For this review, take the finished solid that the model builds, in its own axes (mm). Face numbers are marked on the shaded views. A direction names the side the tool comes from. Give positions to 0.01 mm unless a question says otherwise; leave off trailing zeros. Write each loop counter-clockwise with the first axis right and the second up, starting at its lowest first coordinate (ties: lowest second). Pieces come first, ordered by that corner, then holes. Notation, with made-up numbers: M -3.75,-13 L 24.25,-13 A17 cw 24.25,3 Z; hole C 19,68.5 d6. An arc over 180 degrees is marked long. One line per item, written item: value. Start each with the question number.
Item 1: To check wall thickness, follow probe 1 along Y at (x, z) = (8.5, -13); probe 2 along Y at (x, z) = (26, 10); probe 3 along Z at (x, y) = (-8.5, 2) (3 decimals). State the ranges of each line that lie inside material, in increasing order.
Item 2: Consider section B-B, the plane z = 3. Write out the cut boundary in (x, y), and give its area (3 significant figures).
Item 3: Tool access review of the marked faces 1 and 2: name each direction out of +Z, -Z, +X, -X, +Y, -Y from which nothing blocks a thin tool from reaching the whole face with its end or side.
Item 4: Clearance check with flat-ended pins moving along their axes: pin 1 Ø0.6 at (y, z) = (3, 6.5) entering from +X; pin 2 Ø1 at (x, z) = (3.5, -11) entering from +Y; pin 3 Ø2.5 at (x, z) = (29, -11.875) entering from -Y. State where each tip first meets the part, or that it passes through.
Item 5: Consider section C-C, the plane y = -0.75. Write out the cut boundary in (x, z) (3 decimals), and give its area (3 significant figures).
Item 6: Consider section A-A, the plane x = -0.5. Write out the cut boundary in (y, z) (3 decimals), and give its area (3 significant figures).
```python
from build123d import *

# Parameters (mm, degrees)
EXTRUDE_1_DEPTH     = 1.63
SKETCH_2_R          = 1.5
CUT_EXTRUDE_1_DEPTH = 1.6
SKETCH_3_W          = 26.5
SKETCH_3_H          = 26
EXTRUDE_2_DEPTH     = 1.8
EXTRUDE_3_DEPTH     = 2
SKETCH_4_W          = 5.81
SKETCH_4_H          = 3.67
EXTRUDE_4_DEPTH     = 2
SKETCH_7_W          = 2.6
SKETCH_7_H          = 1.3
EXTRUDE_5_DEPTH     = 1
SKETCH_8_W          = 51
SKETCH_8_H          = 5
EXTRUDE_6_DEPTH     = 3.68
SKETCH_9_W          = 1.9
SKETCH_9_H          = 1.9
EXTRUDE_7_DEPTH     = 3
SKETCH_10_R         = 1.6
EXTRUDE_8_DEPTH     = 1


with BuildPart() as part:
    # 草图1 → 凸台-拉伸1 (new body)
    with BuildSketch(Plane(origin=(0, 0, 0), x_dir=(1, 0, 0), z_dir=(0, 1, 0))):
        with BuildLine():
            Line((-29.5, 15.375), (29.5, 15.375))
            ThreePointArc((29.5, 15.375), (31.621320344, 14.496320344), (32.5, 12.375))
            Line((32.5, 12.375), (32.5, -12.375))
            ThreePointArc((32.5, -12.375), (31.621320344, -14.496320344), (29.5, -15.375))
            Line((29.5, -15.375), (-29.5, -15.375))
            ThreePointArc((-29.5, -15.375), (-31.621320344, -14.496320344), (-32.5, -12.375))
            Line((-32.5, -12.375), (-32.5, 12.375))
            ThreePointArc((-32.5, 12.375), (-31.621320344, 14.496320344), (-29.5, 15.375))
        make_face()
    extrude(amount=EXTRUDE_1_DEPTH)

    # 草图2 → 切除-拉伸1 (cut)
    with BuildSketch(Plane(origin=(0, 1.63, 0), x_dir=(1, 0, 0), z_dir=(0, 1, 0))):
        with Locations(Location((-29, 11.875, 0), (0, 0, 270))):
            Circle(SKETCH_2_R)
        with Locations(Location((-29, -11.875, 0), (0, 0, 270))):
            Circle(SKETCH_2_R)
        with Locations(Location((29, -11.875, 0), (0, 0, 270))):
            Circle(SKETCH_2_R)
        with Locations(Location((29, 11.875, 0), (0, 0, 270))):
            Circle(SKETCH_2_R)
    extrude(amount=-CUT_EXTRUDE_1_DEPTH, mode=Mode.SUBTRACT)

    # 草图3 → 凸台-拉伸2 (add)
    with BuildSketch(Plane(origin=(0, 1.63, 0), x_dir=(1, 0, 0), z_dir=(0, 1, 0))):
        with Locations((1.45, -0.075)):
            Rectangle(SKETCH_3_W, SKETCH_3_H)
    extrude(amount=EXTRUDE_2_DEPTH)

    # 草图5 → 凸台-拉伸3 (add)
    with BuildSketch(Plane(origin=(0, 1.63, 0), x_dir=(1, 0, 0), z_dir=(0, 1, 0))):
        with BuildLine():
            Line((27.074695167, 3.918250353), (29.514213562, 1.478731957))
            ThreePointArc((29.514213562, 1.478731957), (30.1, 0.064518395), (29.514213562, -1.349695167))
            Line((29.514213562, -1.349695167), (27.074695167, -3.789213562))
            ThreePointArc((27.074695167, -3.789213562), (25.660481605, -4.375), (24.246268043, -3.789213562))
            Line((24.246268043, -3.789213562), (21.806749647, -1.349695167))
            ThreePointArc((21.806749647, -1.349695167), (21.22096321, 0.064518395), (21.806749647, 1.478731957))
            Line((21.806749647, 1.478731957), (24.246268043, 3.918250353))
            ThreePointArc((24.246268043, 3.918250353), (25.660481605, 4.50403679), (27.074695167, 3.918250353))
        make_face()
    extrude(amount=EXTRUDE_3_DEPTH)

    # 草图4 → 凸台-拉伸4 (add)
    with BuildSketch(Plane(origin=(0, 1.63, 0), x_dir=(1, 0, 0), z_dir=(0, 1, 0))):
        with Locations((-24.325, 6.45)):
            Rectangle(SKETCH_4_W, SKETCH_4_H)
        with Locations((-24.325, 0.18)):
            Rectangle(SKETCH_4_W, SKETCH_4_H)
        with Locations((-24.325, -6.09)):
            Rectangle(SKETCH_4_W, SKETCH_4_H)
    extrude(amount=EXTRUDE_4_DEPTH)

    # 草图7 → 凸台-拉伸5 (add)
    with BuildSketch(Plane(origin=(0, 3.63, 0), x_dir=(1, 0, 0), z_dir=(0, 1, 0))):
        with Locations((-24.325, 6.45)):
            Rectangle(SKETCH_7_W, SKETCH_7_H)
        with Locations((-24.325, 0.18)):
            Rectangle(SKETCH_7_W, SKETCH_7_H)
        with Locations((-24.325, -6.09)):
            Rectangle(SKETCH_7_W, SKETCH_7_H)
    extrude(amount=EXTRUDE_5_DEPTH)

    # 草图8 → 凸台-拉伸6 (add)
    with BuildSketch(Plane.XZ):
        with Locations((-0.2, -11.235)):
            Rectangle(SKETCH_8_W, SKETCH_8_H)
    extrude(amount=EXTRUDE_6_DEPTH)

    # 草图9 → 凸台-拉伸7 (add)
    with BuildSketch(Plane(origin=(0, 3.63, 0), x_dir=(1, 0, 0), z_dir=(0, 1, 0))):
        with Locations((25.660481605, 0.064518395)):
            Rectangle(SKETCH_9_W, SKETCH_9_H)
    extrude(amount=EXTRUDE_7_DEPTH)

    # 草图10 → 凸台-拉伸8 (add)
    with BuildSketch(Plane(origin=(0, 3.63, 0), x_dir=(1, 0, 0), z_dir=(0, 1, 0))):
        with Locations(Location((25.660481605, 0.064518395, 0), (0, 0, 90))):
            Circle(SKETCH_10_R)
    extrude(amount=EXTRUDE_8_DEPTH)


solid = part.part
```
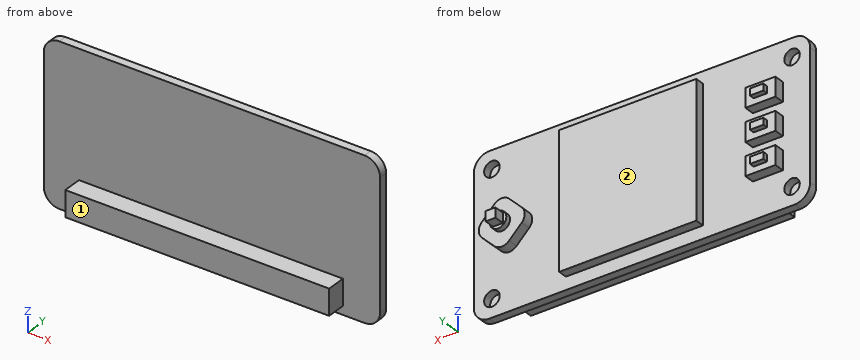
Model answer:
1. probe 1: y = -3.68 to 1.63
1. probe 2: y = 0 to 1.63
1. probe 3: z = -12.925 to 13.075
2. outline: M -32.5,0 L 32.5,0 L 32.5,1.63 L 27.86,1.63 L 27.86,3.63 L 23.46,3.63 L 23.46,1.63 L 14.7,1.63 L 14.7,3.43 L -11.8,3.43 L -11.8,1.63 L -32.5,1.63 Z
2. area: 162 mm2
3. face 1: +Z, -Z, +X, -X, -Y
3. face 2: +Z, -Z, +Y
4. pin 1: stops at x = 14.7
4. pin 2: stops at y = 3.43
4. pin 3: stops at y = 0
5. outline: M -25.7,-13.735 L 25.3,-13.735 L 25.3,-8.735 L -25.7,-8.735 Z
5. area: 255 mm2
6. outline: M -3.68,-13.735 L 0,-13.735 L 0,-15.375 L 1.63,-15.375 L 1.63,-12.925 L 3.43,-12.925 L 3.43,13.075 L 1.63,13.075 L 1.63,15.375 L 0,15.375 L 0,-8.735 L -3.68,-8.735 Z
6. area: 115 mm2
